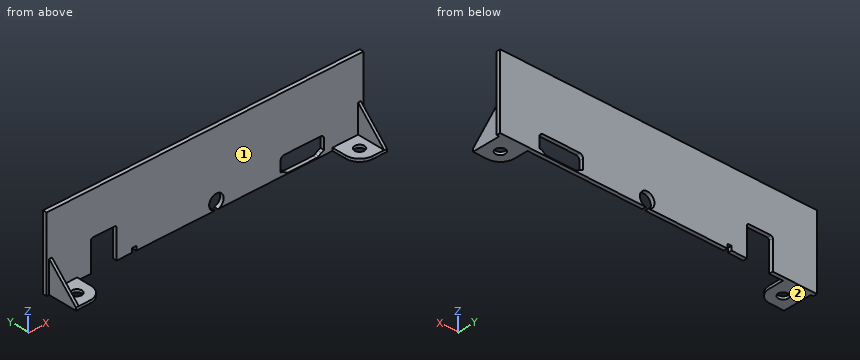
from build123d import *

# Parameters (mm, degrees)
PAD028_DEPTH    = 1.4
SKETCH048_R     = 1.75
PAD029_DEPTH    = 1
PAD030_DEPTH    = 1
PAD031_DEPTH    = 1
SKETCH179_W     = 1.5
SKETCH179_H     = 1.5
POCKET061_DEPTH = 5


with BuildPart() as part:
    # Sketch047 (on Face725 of Binder021) → Pad028 (new body)
    with BuildSketch(Plane(origin=(0, 135.8, 0), x_dir=(-1, 0, 0), z_dir=(0, 1, 0))):
        with BuildLine():
            Line((-120.499982, -0.1), (-120.499982, -26.3))
            Line((-120.499982, -26.3), (-68.48194, -26.3))
            ThreePointArc((-67.46705, -26.3), (-67.974495, -21.15), (-68.48194, -26.3))
            Line((-67.46705, -26.3), (-32.299995, -26.3))
            Line((-32.299995, -15.934266), (-32.299995, -26.3))
            ThreePointArc((-31.615729, -15.25), (-32.099578, -15.450417), (-32.299995, -15.934266))
            Line((-31.615729, -15.25), (-23.784261, -15.25))
            ThreePointArc((-23.099995, -15.934266), (-23.300412, -15.450417), (-23.784261, -15.25))
            Line((-23.099995, -15.934266), (-23.099995, -26.3))
            Line((-7.299995, -26.3), (-23.099995, -26.3))
            Line((-7.299995, -26.3), (-7.299995, -0.1))
            Line((-7.299995, -0.1), (-120.499982, -0.1))
        make_face()
        with BuildLine():
            Line((-105.199995, -19.86), (-92.199994, -19.86))
            ThreePointArc((-90.899995, -21.16), (-91.280756, -20.240762), (-92.199994, -19.86))
            Line((-90.899995, -21.16), (-90.899995, -24.776619))
            Line((-90.899995, -24.776619), (-91.938732, -25.120886))
            Line((-91.938732, -25.120886), (-92.869018, -25.773985))
            ThreePointArc((-93.61597, -26.01), (-93.224294, -25.949593), (-92.869018, -25.773985))
            Line((-93.61597, -26.01), (-103.78402, -26.01))
            ThreePointArc((-104.530977, -25.773981), (-104.175699, -25.949592), (-103.78402, -26.01))
            Line((-105.461258, -25.120886), (-104.530977, -25.773981))
            Line((-106.499995, -24.776619), (-105.461258, -25.120886))
            Line((-106.499995, -21.16), (-106.499995, -24.776619))
            ThreePointArc((-105.199995, -19.86), (-106.119234, -20.240761), (-106.499995, -21.16))
        make_face(mode=Mode.SUBTRACT)
    extrude(amount=-PAD028_DEPTH)

    # Sketch048 (on Face5 of Binder022) → Pad029 (join)
    with BuildSketch(Plane.XY.offset(-26.3)):
        with BuildLine():
            Line((18.199995, 134.4), (8.199995, 134.4))
            Line((8.199995, 134.4), (8.199995, 124.1))
            Line((8.199995, 124.1), (13.199995, 124.1))
            ThreePointArc((13.199995, 124.1), (16.735529, 125.564466), (18.199995, 129.1))
            Line((18.199995, 134.4), (18.199995, 129.1))
        make_face()
        with Locations((13.199995, 129.1)):
            Circle(SKETCH048_R, mode=Mode.SUBTRACT)
        with BuildLine():
            Line((109.449995, 134.4), (119.599982, 134.4))
            Line((119.599982, 134.4), (119.599982, 124.35))
            Line((119.599982, 124.35), (114.449995, 124.35))
            ThreePointArc((109.449995, 129.35), (110.914461, 125.814466), (114.449995, 124.35))
            Line((109.449995, 134.4), (109.449995, 129.35))
        make_face()
        with Locations((114.449995, 129.35)):
            Circle(SKETCH048_R, mode=Mode.SUBTRACT)
    extrude(amount=PAD029_DEPTH)

    # Sketch049 (on Face25 of Pad029) → Pad030 (join)
    with BuildSketch(Plane(origin=(8.199995, 0, 0), x_dir=(0, -1, 0), z_dir=(-1, 0, 0))):
        Polygon((-134.4, -25.3), (-124.1, -25.3), (-134.4, -15), align=None)
    extrude(amount=-PAD030_DEPTH)

    # Sketch050 (on Face36 of Pad030) → Pad031 (join)
    with BuildSketch(Plane.YZ.offset(119.599982)):
        Polygon((124.35, -25.3), (134.4, -25.3), (134.4, -15.25), align=None)
    extrude(amount=-PAD031_DEPTH)

    # Sketch179 (on Face4 of Clone005) → Pocket061 (cut)
    with BuildSketch(Plane(origin=(0, 135.8, 0), x_dir=(-1, 0, 0), z_dir=(0, 1, 0))):
        with Locations((-38.579995, -25.55)):
            Rectangle(SKETCH179_W, SKETCH179_H)
    extrude(amount=-POCKET061_DEPTH, mode=Mode.SUBTRACT)


solid = part.part
Design review of the part built by this model. Coordinates are the model's own, in mm. Face numbers are marked on the shaded views. Round coordinates to 2 decimals unless told otherwise and drop trailing zeros. Write each loop counter-clockwise with the first axis right and the second up, starting at its lowest first coordinate (ties: lowest second). Pieces come first, ordered by that corner, then holes. Notation, with made-up numbers: (57.5, 52) - (77.5, 52) arc R24 cw to (77.5, 71) - close; hole circle Ø4 at (33, -1.75). An arc over 180 degrees is marked (long way). Use a Markdown table: item, result. Add a question column.
1. We need section D-D (x = 111.5). State the section outline as (y, z) points.
2. We need section C-C (z = -8.25). State the section outline as (x, y) points.
3. We need section B-B (x = 43.5). State the section outline as (y, z) points, then the cut area to 3 significant figures.
4. Wall thickness on probe 1 along X at (y, z) = (135.25, -23.75); probe 2 along X at (y, z) = (129.1, -26); probe 3 along X at (y, z) = (134, -23): over which ranges is each line inside the solid? List them lowest first.
5. We need section A-A (z = -23.75). State the section outline as (x, y) points, then the cut area to 3 significant figures.
6. Mouldability with a two-part tool opening along X and no side actions: class the marked faces 1 and 2 as +X half, -X half, draft (parallel to the pull), parting line (faces both ways), or undercut.
7. Clearance check with flat-ended pins moving along their axes: pin 1 (6 mm diameter, centred on x = 54.5, y = 130, fed in from +Z); pin 2 (4 mm diameter, centred on y = 130.5, z = -23.5, fed in from -X); pin 3 (1.1 mm diameter, centred on y = 132, z = -25.5, fed in from +X); pin 4 (4 mm diameter, centred on x = 72, z = -18.5, fed in from -Y). State where each tip first meets the part, or that it passes through.
Output:
| question | item | result |
|---|---|---|
| 1 | outline | (125.31, -26.3) - (135.8, -26.3) - (135.8, -0.1) - (134.4, -0.1) - (134.4, -25.3) - (125.31, -25.3) - close |
| 2 | outline | (7.3, 134.4) - (120.5, 134.4) - (120.5, 135.8) - (7.3, 135.8) - close |
| 3 | outline | (134.4, -26.3) - (135.8, -26.3) - (135.8, -0.1) - (134.4, -0.1) - close |
| 3 | area | 36.7 mm2 |
| 4 | probe 1 | x = 7.3 to 23.1, 32.3 to 65.37, 70.57 to 90.9, 106.5 to 120.5 |
| 4 | probe 2 | x = 8.2 to 11.45, 14.95 to 18.2, 109.46 to 112.72, 116.18 to 119.6 |
| 4 | probe 3 | x = 8.2 to 9.2, 118.6 to 119.6 |
| 5 | outline | (7.3, 134.4) - (8.2, 134.4) - (8.2, 125.65) - (9.2, 125.65) - (9.2, 134.4) - (23.1, 134.4) - (23.1, 135.8) - (7.3, 135.8) - close; (32.3, 134.4) - (65.37, 134.4) - (65.37, 135.8) - (32.3, 135.8) - close; (70.57, 134.4) - (90.9, 134.4) - (90.9, 135.8) - (70.57, 135.8) - close; (106.5, 134.4) - (118.6, 134.4) - (118.6, 125.9) - (119.6, 125.9) - (119.6, 134.4) - (120.5, 134.4) - (120.5, 135.8) - (106.5, 135.8) - close |
| 5 | area | 134 mm2 |
| 6 | face 1 | undercut |
| 6 | face 2 | draft |
| 7 | pin 1 | passes through |
| 7 | pin 2 | stops at x = 8.2 |
| 7 | pin 3 | stops at x = 119.6 |
| 7 | pin 4 | stops at y = 134.4 |
